```python
from build123d import *

# Parameters (mm, degrees)
BOSS_EXTRUDE1_START = 4
SKETCH1_W           = 104.9
SKETCH1_H           = 168.1
BOSS_EXTRUDE1_DEPTH = 1
SKETCH2_W           = 8.9
SKETCH2_H           = 25
BOSS_EXTRUDE2_DEPTH = 4
SKETCH5_R           = 2.1
CUT_EXTRUDE5_DEPTH  = 6
CUT_EXTRUDE3_REACH  = 7
SKETCH3_R           = 1.475
SKETCH3_W           = 15.52
SKETCH3_H           = 20.32
FILLET1_R           = 2


with BuildPart() as part:
    # Sketch1 → Boss-Extrude1 (new body)
    with BuildSketch(Plane.XY.offset(BOSS_EXTRUDE1_START)):
        with Locations((52.45, -16.15)):
            Rectangle(SKETCH1_W, SKETCH1_H)
    extrude(amount=BOSS_EXTRUDE1_DEPTH)

    # Sketch2 → Boss-Extrude2 (add)
    with BuildSketch(Plane(origin=(0, 0, 4), x_dir=(-1, 0, 0), z_dir=(0, 0, -1))):
        with Locations((-100.45, 33.95)):
            Rectangle(SKETCH2_W, SKETCH2_H)
        with Locations((-4.45, 33.95)):
            Rectangle(SKETCH2_W, SKETCH2_H)
        with Locations((-4.45, -66.25)):
            Rectangle(SKETCH2_W, SKETCH2_H)
        with Locations((-100.45, -66.25)):
            Rectangle(SKETCH2_W, SKETCH2_H)
    extrude(amount=BOSS_EXTRUDE2_DEPTH)

    # Sketch5 → Cut-Extrude5 (cut, through all)
    with BuildSketch(Plane.XY.offset(5)):
        with Locations((100.45, -74.25)):
            Circle(SKETCH5_R)
        with Locations((100.45, -58.25)):
            Circle(SKETCH5_R)
        with Locations((4.45, -74.25)):
            Circle(SKETCH5_R)
        with Locations((4.45, -58.25)):
            Circle(SKETCH5_R)
        with Locations((4.45, 25.95)):
            Circle(SKETCH5_R)
        with Locations((4.45, 41.95)):
            Circle(SKETCH5_R)
        with Locations((100.45, 25.95)):
            Circle(SKETCH5_R)
        with Locations((100.45, 41.95)):
            Circle(SKETCH5_R)
    extrude(amount=-CUT_EXTRUDE5_DEPTH, mode=Mode.SUBTRACT)

    # Sketch3 → Cut-Extrude3 (cut, up to next)
    with BuildSketch(Plane.XY.offset(5), mode=Mode.PRIVATE) as cut_extrude3_sk1:
        with Locations((44.661, 26.076)):
            Circle(SKETCH3_R)
    cut_extrude3_tool1 = extrude(cut_extrude3_sk1.sketch, amount=-CUT_EXTRUDE3_REACH, mode=Mode.PRIVATE) & part.part
    add(cut_extrude3_tool1.solids().sort_by_distance((44.661, 26.076, 5))[0], mode=Mode.SUBTRACT)
    # Sketch3 → Cut-Extrude3 (cut, up to next)
    with BuildSketch(Plane.XY.offset(5), mode=Mode.PRIVATE) as cut_extrude3_sk2:
        with Locations((44.661, 41.316)):
            Circle(SKETCH3_R)
    cut_extrude3_tool2 = extrude(cut_extrude3_sk2.sketch, amount=-CUT_EXTRUDE3_REACH, mode=Mode.PRIVATE) & part.part
    add(cut_extrude3_tool2.solids().sort_by_distance((44.661, 41.316, 5))[0], mode=Mode.SUBTRACT)
    # Sketch3 → Cut-Extrude3 (cut, up to next)
    with BuildSketch(Plane.XY.offset(5), mode=Mode.PRIVATE) as cut_extrude3_sk3:
        with Locations((54.596, 33.696)):
            Rectangle(SKETCH3_W, SKETCH3_H)
    cut_extrude3_tool3 = extrude(cut_extrude3_sk3.sketch, amount=-CUT_EXTRUDE3_REACH, mode=Mode.PRIVATE) & part.part
    add(cut_extrude3_tool3.solids().sort_by_distance((54.596, 33.696, 5))[0], mode=Mode.SUBTRACT)

    # Fillet1
    fillet1_edges = [part.edges().sort_by_distance(p)[0] for p in [
        (0, 67.9, 4.5),
        (104.9, 67.9, 4.5),
        (104.9, -100.2, 4.5),
        (0, -100.2, 4.5),
    ]]
    fillet(fillet1_edges, radius=FILLET1_R)


solid = part.part
```
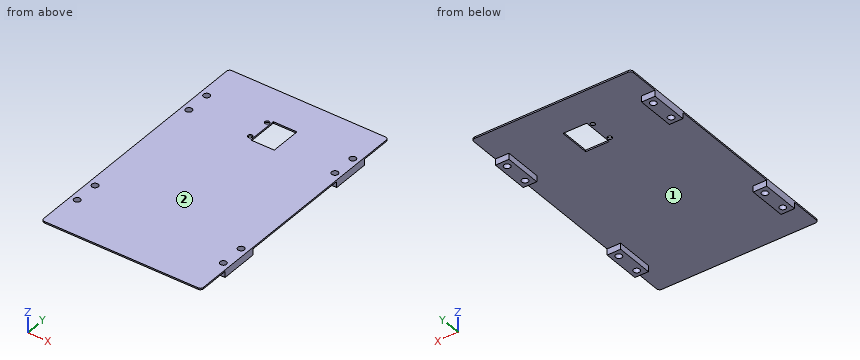
Input: part model. Units: mm. Frame: model coordinates. Face numbers are marked on the shaded views. Give positions to 0.01 mm unless a question says otherwise; leave off trailing zeros. Order: outer loops, then holes, each group sorted by start corner. A loop starts at its lowest first (then second) coordinate and runs counter-clockwise, first axis right, second up. Notation, with made-up numbers: M -38,51.25 L 16,51.25 A29 ccw 16,89.25 Z; hole C 87,36 d3. An arc over 180 degrees is marked long. One line per question, with ' | ' between items. Start each with the question number.
1. First-contact query: pin 1 Ø8 at (x, y) = (64.5, -47.5) entering from -Z; pin 2 Ø2.5 at (x, y) = (100.45, 25.95) entering from -Z; pin 3 Ø3 at (x, z) = (6.5, 2) entering from -Y. Flat tips, straight axial feed; report the tip coordinate or a pass-through.
2. Section query B-B (y = -58.25). Return the cut outline in (x, z).
3. Section query D-D (y = 15). Return the cut outline in (x, z), and give its area (3 significant figures).
4. Pull-direction query (X, two-part tool) for the marked faces 1 and 2; classes: released by +X, released by -X, zero draft, split by the parting line, or undercut.
5. Section query A-A (z = 3.15). Count the separate pieces of the cut face and the enclosed holes in it, and give its area (3 significant figures).
6. Material intervals for probe 1 along Y at (x, z) = (4.45, 3.05); probe 2 along Y at (x, z) = (8.5, 2.8); probe 3 along Y at (x, z) = (45.5, 4.2), sorted ascending. Write a range as [from, to].
7. Section query C-C (x = 53). Return the cut outline in (y, z).
Here are the results:
1) pin 1: z = 4 | pin 2: through | pin 3: y = -78.75
2) outline: M 0,0 L 2.35,0 L 2.35,5 L 0,5 Z; M 6.55,0 L 8.9,0 L 8.9,4 L 96,4 L 96,0 L 98.35,0 L 98.35,5 L 6.55,5 Z; M 102.55,0 L 104.9,0 L 104.9,5 L 102.55,5 Z
3) outline: M 0,4 L 104.9,4 L 104.9,5 L 0,5 Z | area: 105 mm²
4) face 1: undercut | face 2: zero draft
5) separate pieces: 4 | enclosed holes: 8 | area: 779 mm²
6) probe 1: [-78.75, -76.35], [-72.15, -60.35], [-56.15, -53.75], [21.45, 23.85], [28.05, 39.85], [44.05, 46.45] | probe 2: [-78.75, -53.75], [21.45, 46.45] | probe 3: [-100.2, 24.86], [27.29, 40.1], [42.53, 67.9]
7) outline: M -100.2,4 L 23.54,4 L 23.54,5 L -100.2,5 Z; M 43.86,4 L 67.9,4 L 67.9,5 L 43.86,5 Z
